```python
from build123d import *

# Parameters (mm, degrees)
SKETCH3_W                       = 63.5
SKETCH3_H                       = 2.286
BASE_FLANGE1_DEPTH              = 31.75
FILLET1_R                       = 2.54
F_25_0_1495_DIAMETER_HOLE1_D    = 3.7973
SKETCH10_R                      = 11.43
CUT_EXTRUDE1_DEPTH              = 45.959435005
F_7_32_0_21875_DIAMETER_HOLE1_D = 5.55625
F_1_8_0_125_DIAMETER_HOLE1_D    = 3.175


# Sheet-metal steps are written as plain solids
with BuildPart() as part:
    # Sketch3 → Base-Flange1 (new, symmetric)
    with BuildSketch(Plane(origin=(0, 0, 0), x_dir=(-1, 0, 0), z_dir=(0, 1, 0))):
        with Locations((0, -1.143)):
            Rectangle(SKETCH3_W, SKETCH3_H)
    extrude(amount=BASE_FLANGE1_DEPTH, both=True)

    # Fillet1
    fillet1_edges = [part.edges().sort_by_distance(p)[0] for p in [
        (31.75, 31.75, -1.143),
        (31.75, -31.75, -1.143),
        (-31.75, -31.75, -1.143),
        (-31.75, 31.75, -1.143),
    ]]
    fillet(fillet1_edges, radius=FILLET1_R)

    # #25 (0.1495) Diameter Hole1 (through all)
    with Locations(Plane.XY):
        with Locations((-25.4, 19.05), (25.4, 19.05), (25.4, -19.05), (-25.4, -19.05)):
            Hole(F_25_0_1495_DIAMETER_HOLE1_D / 2)

    # Sketch10 → Cut-Extrude1 (cut, through all)
    with BuildSketch(Plane.XY):
        Circle(SKETCH10_R)
    extrude(amount=-CUT_EXTRUDE1_DEPTH, mode=Mode.SUBTRACT)

    # 7/32 (0.21875) Diameter Hole1 (through all)
    with Locations(Plane.XY):
        with Locations((25.4, 0)):
            Hole(F_7_32_0_21875_DIAMETER_HOLE1_D / 2)

    # 1/8 (0.125) Diameter Hole1 (through all)
    with Locations(Plane.XY):
        with Locations((0, 16), (0, -16)):
            Hole(F_1_8_0_125_DIAMETER_HOLE1_D / 2)


solid = part.part
```
Model file for the job. Use its own axes, mm. Coordinates: 2 decimals unless noted, no trailing zeros. Loops run counter-clockwise (first coordinate to the right, second up) from the corner with the lowest first, then second, coordinate; pieces in that order, holes last. Notation, with made-up numbers: (59.25, -18) - (66.25, -18) arc R6 cw to (66.25, -9) - close; hole circle Ø10 at (49.25, 9.25). An arc over 180 degrees is marked (long way). Write item = value, one per line. Start each with the question number.
Item 1: Saw through at A-A, the plane y = 0. List the corners of the cut face in (x, z).
Item 2: Saw through at B-B, the plane z = -1.8. State how many separate pieces and enclosed holes the cut face has, then the cut area to 3 significant figures.
Item 3: Saw through at C-C, the plane x = -25.4. List the corners of the cut face in (y, z).
Item 4: Saw through at D-D, the plane y = -16. List the corners of the cut face in (x, z), then the cut area to 3 significant figures.
Item 5: Wall check: probe 1 along Y at (x, z) = (0, -0.6); probe 2 along Y at (x, z) = (25.4, -1.1); probe 3 along Y at (x, z) = (-25.4, -1.45). Give the ranges that are in metal, low to high. Write a range as [from, to].
Item 6: Pull direction Y, two halves, no side cores. Call faces 1 (the face through (-24.988, 17.196, -1.159)), 2 (the face through (0, -14, 0)), 3 (the face through (-31.026, -30.986, -1.127)): +Y half, -Y half, draft (parallel to the pull), parting line (faces both ways), or undercut.
Answers:
q1.outline = (-31.75, -2.29) - (-11.43, -2.29) - (-11.43, 0) - (-31.75, 0) - close; (11.43, -2.29) - (22.62, -2.29) - (22.62, 0) - (11.43, 0) - close; (28.18, -2.29) - (31.75, -2.29) - (31.75, 0) - (28.18, 0) - close
q2.separate_pieces = 1
q2.enclosed_holes = 8
q2.area = 3,530 mm2
q3.outline = (-31.75, -2.29) - (-20.95, -2.29) - (-20.95, 0) - (-31.75, 0) - close; (-17.15, -2.29) - (17.15, -2.29) - (17.15, 0) - (-17.15, 0) - close; (20.95, -2.29) - (31.75, -2.29) - (31.75, 0) - (20.95, 0) - close
q4.outline = (-31.75, -2.29) - (-1.59, -2.29) - (-1.59, 0) - (-31.75, 0) - close; (1.59, -2.29) - (31.75, -2.29) - (31.75, 0) - (1.59, 0) - close
q4.area = 138 mm2
q5.probe_1 = [-31.75, -17.59], [-14.41, -11.43], [11.43, 14.41], [17.59, 31.75]
q5.probe_2 = [-31.75, -20.95], [-17.15, -2.78], [2.78, 17.15], [20.95, 31.75]
q5.probe_3 = [-31.75, -20.95], [-17.15, 17.15], [20.95, 31.75]
q6.face_1 = undercut
q6.face_2 = draft
q6.face_3 = -Y half
